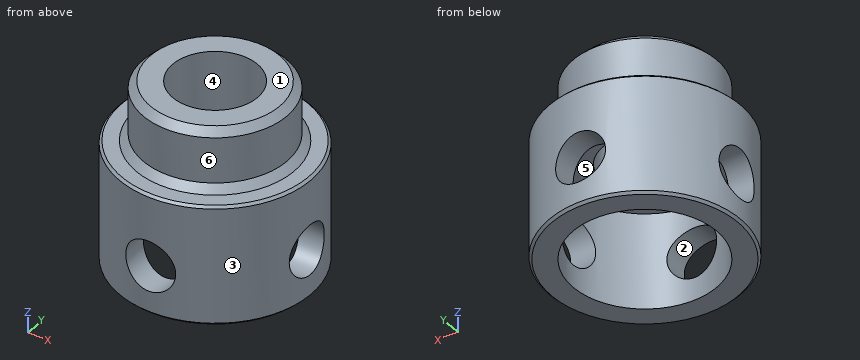
from build123d import *

# Parameters (mm, degrees)
SKETCH_R        = 8
PAD_DEPTH       = 10
SKETCH001_R     = 6
PAD001_DEPTH    = 5
SKETCH002_R     = 3.55
POCKET_DEPTH    = 20
SKETCH003_R     = 6
POCKET001_DEPTH = 8
SKETCH004_R     = 2.1
POCKET002_DEPTH = 50
SKETCH005_R     = 2.1
POCKET003_DEPTH = 50
CHAMFER_SIZE    = 0.6
CHAMFER001_SIZE = 0.2
CHAMFER002_SIZE = 0.2


with BuildPart() as part:
    # Sketch → Pad (new body)
    with BuildSketch(Plane.XY):
        Circle(SKETCH_R)
    extrude(amount=PAD_DEPTH)

    # Sketch001 (on Face3 of Pad) → Pad001 (join)
    with BuildSketch(Plane.XY.offset(10)):
        Circle(SKETCH001_R)
    extrude(amount=PAD001_DEPTH)

    # Sketch002 (on Face5 of Pad001) → Pocket (cut)
    with BuildSketch(Plane.XY.offset(15)):
        Circle(SKETCH002_R)
    extrude(amount=-POCKET_DEPTH, mode=Mode.SUBTRACT)

    # Sketch003 (on Face2 of Pocket) → Pocket001 (cut)
    with BuildSketch(Plane(origin=(0, 0, 0), x_dir=(1, 0, 0), z_dir=(0, 0, -1))):
        Circle(SKETCH003_R)
    extrude(amount=-POCKET001_DEPTH, mode=Mode.SUBTRACT)

    # Sketch004 → Pocket002 (cut, symmetric)
    with BuildSketch(Plane.XZ):
        with Locations((0, 4)):
            Circle(SKETCH004_R)
    extrude(amount=POCKET002_DEPTH, both=True, mode=Mode.SUBTRACT)

    # Sketch005 → Pocket003 (cut, symmetric)
    with BuildSketch(Plane.YZ):
        with Locations((0, 4)):
            Circle(SKETCH005_R)
    extrude(amount=POCKET003_DEPTH, both=True, mode=Mode.SUBTRACT)

    # Chamfer
    chamfer_edges = [part.edges().sort_by_distance(p)[0] for p in [
        (6, 0, 12.5),
        (-6, 0, 10),
        (-6, 0, 15),
    ]]
    chamfer(chamfer_edges, length=CHAMFER_SIZE)

    # Chamfer001
    chamfer001_edges = [part.edges().sort_by_distance(p)[0] for p in [
        (-8, 0, 10),
    ]]
    chamfer(chamfer001_edges, length=CHAMFER001_SIZE)

    # Chamfer002
    chamfer002_edges = [part.edges().sort_by_distance(p)[0] for p in [
        (-8, 0, 0),
    ]]
    chamfer(chamfer002_edges, length=CHAMFER002_SIZE)


solid = part.part
CAD build for the part. Positions are in the model's coordinates, mm. Face numbers are marked on the shaded views. A direction names the side the tool comes from. Round coordinates to 2 decimals unless told otherwise and drop trailing zeros. Order: outer loops, then holes, each group sorted by start corner. A loop starts at its lowest first (then second) coordinate and runs counter-clockwise, first axis right, second up. Notation, with made-up numbers: (14, -37.5) -> (18, -37.5) arc R15 ccw to (18, -28.5) -> close; hole circle Ø4 at (48, 0.25). An arc over 180 degrees is marked (long way). Write item = value, one per line. Start each with the question number.
(1) Which spindle directions (+Z, -Z, +X, -X, +Y, -Y) get a long thin tool onto all of the face, cutting with end or side? Do the marked faces 4, 5 and 6. Say none if no direction does.
(2) Cut at C-C, the plane z = 4. List the corners of the cut face in (x, y).
(3) Pull direction X, two halves, no side cores. Call the marked faces 1, 2 and 3: released by +X, released by -X, zero draft, split by the parting line, or undercut.
(4) Probe line 1 (Z direction, x = 6.9, y = 0); line 2 (Y direction, x = -3, z = 13.75); line 3 (Y direction, x = -0.75, z = 6). List the from-to ranges inside material, lowest first. Write a range as [from, to].
(5) Pin check, flat tips, straight feed: P1, Ø3, axis at x = 6, z = 9, coming from the +Y side; P2, Ø4, axis at x = 0, z = 4, coming from the -Y side; P3, Ø1, axis at x = 5, z = 11, coming from the -Y side. Stop position of each tip, or through.
(6) Cut at A-A, the plane x = 0. State how many separate pieces and enclosed holes the cut face has, then the cut area to 3 significant figures.
(7) Cut at D-D, the plane z = 11. List the corners of the cut face in (x, y).
Model answer:
q1.face_4 = +Z, -Z
q1.face_5 = -Z
q1.face_6 = +Z
q2.outline = (-7.72, -2.1) arc R8 ccw to (-2.1, -7.72) -> (-2.1, -5.62) arc R6 cw to (-5.62, -2.1) -> close; (-7.72, 2.1) -> (-5.62, 2.1) arc R6 cw to (-2.1, 5.62) -> (-2.1, 7.72) arc R8 ccw to start; (2.1, -7.72) arc R8 ccw to (7.72, -2.1) -> (5.62, -2.1) arc R6 cw to (2.1, -5.62) -> close; (2.1, 5.62) arc R6 cw to (5.62, 2.1) -> (7.72, 2.1) arc R8 ccw to (2.1, 7.72) -> close
q3.face_1 = zero draft
q3.face_2 = undercut
q3.face_3 = split by the parting line
q4.line_1 = [0, 1.9], [6.1, 10]
q4.line_2 = [-5.2, -1.9], [1.9, 5.2]
q4.line_3 = [-7.96, -5.95], [5.95, 7.96]
q5.P1 = 6.61
q5.P2 = through
q5.P3 = -3.97
q6.separate_pieces = 4
q6.enclosed_holes = 0
q6.area = 57.4 mm2
q7.outline = circle Ø12 at (0, 0); hole circle Ø7.1 at (0, 0)
